from build123d import *

# Parameters (mm, degrees)
CUT_EXTRUDE_1_DEPTH      = 6
CUT_EXTRUDE_1_DEPTH_BACK = 6
SKETCH_2_W               = 26
SKETCH_2_H               = 10


with BuildPart() as part:
    # Sketch 1 → Revolve 1 (revolve)
    with BuildSketch(Plane.XY, mode=Mode.PRIVATE) as revolve_1_sk:
        Polygon((0, 0), (170, 0), (170, 10), (150, 10), (150, 15), (80, 15), (80, 20), (50, 20), (50, 12.5), (0, 12.5), align=None)
    revolve(revolve_1_sk.sketch.rotate(Axis((-10, 0, 0), (1, 0, 0)), 90), axis=Axis((-10, 0, 0), (1, 0, 0)))

    # Sketch 2 → Cut-Extrude 1 (cut, two sides: drawn at the far end of the back side and taken through both)
    with BuildSketch(Plane.XY.offset(-CUT_EXTRUDE_1_DEPTH_BACK)):
        with Locations((65, 20)):
            Rectangle(SKETCH_2_W, SKETCH_2_H)
    extrude(amount=CUT_EXTRUDE_1_DEPTH + CUT_EXTRUDE_1_DEPTH_BACK, mode=Mode.SUBTRACT)


solid = part.part
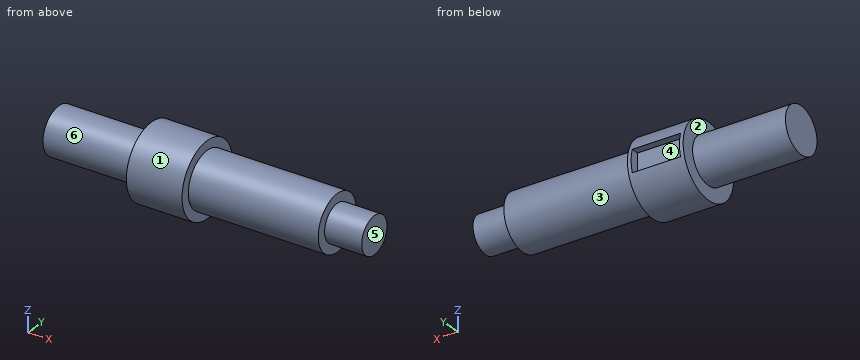
The listing builds one solid part. Answer for the finished solid, in the listing's coordinates (mm). Face numbers are marked on the shaded views. A direction names the side the tool comes from. Coordinates: 2 decimals unless noted, no trailing zeros. Write each loop counter-clockwise with the first axis right and the second up, starting at its lowest first coordinate (ties: lowest second). Pieces come first, ordered by that corner, then holes. Notation, with made-up numbers: (78.5, 86.5) - (86.5, 86.5) arc R23 cw to (86.5, 100.5) - close; hole circle Ø1 at (-14.75, 67). An arc over 180 degrees is marked (long way). Put each result on its own line as item: value.
1. Find the intervals of material crossed by line 1 along X through (y, z) = (-12, 3); line 2 along Z through (x, y) = (146.5, -0.5); line 3 along X through (y, z) = (18, -8), in increasing order. Write a range as from..to.
Answer sheet:
line 1: x = 0..150
line 2: z = -14.99..14.99
line 3: x = 50..80
2. The part is cut by section B-B on z = 0. Give the vertices of the cut face in (x, y), plus the area to 3 significant figures.
Answer sheet:
outline: (0, -12.5) - (50, -12.5) - (50, -20) - (80, -20) - (80, -15) - (150, -15) - (150, -10) - (170, -10) - (170, 10) - (150, 10) - (150, 15) - (80, 15) - (80, 20) - (78, 20) - (78, 15) - (52, 15) - (52, 20) - (50, 20) - (50, 12.5) - (0, 12.5) - close
area: 4,820 mm^2
3. Flat-ended cylindrical pins translate along their axes: pin 1 Ø1 at (x, y) = (147, 2.5) entering from +Z; pin 2 Ø1.5 at (y, z) = (-11.5, -13) entering from -X; pin 3 Ø6 at (x, z) = (67, 1) entering from +Y. Find the tip coordinate at first contact, or state that the pin passes through.
Answer sheet:
pin 1: stops at z = 14.87
pin 2: stops at x = 50
pin 3: stops at y = 15
4. The part is cut by section D-D on z = -8. Give the vertices of the cut face in (x, y).
Answer sheet:
outline: (0, -9.6) - (50, -9.6) - (50, -18.33) - (80, -18.33) - (80, -12.69) - (150, -12.69) - (150, -6) - (170, -6) - (170, 6) - (150, 6) - (150, 12.69) - (80, 12.69) - (80, 18.33) - (50, 18.33) - (50, 9.6) - (0, 9.6) - close
5. The part is cut by section C-C on x = 65. Give the vertices of the cut face in (y, z).
Answer sheet:
outline: (15, -6) - (15, 6) - (19.08, 6) arc R20 ccw (long way) to (19.08, -6) - close
6. The part is cut by section A-A on y = 0. Give the vertices of the cut face in (x, z), plus the area to 3 significant figures.
Answer sheet:
outline: (0, -12.5) - (50, -12.5) - (50, -20) - (80, -20) - (80, -15) - (150, -15) - (150, -10) - (170, -10) - (170, 10) - (150, 10) - (150, 15) - (80, 15) - (80, 20) - (50, 20) - (50, 12.5) - (0, 12.5) - close
area: 4,950 mm^2
7. Determine the mould class of the marked faces 4, 5 and 6 for opening direction Y: pulls with the +Y half, pulls with the -Y half, needs draft (parallel to the pull), parting line crosses it, or undercut.
Answer sheet:
face 4: pulls with the +Y half
face 5: needs draft
face 6: parting line crosses it
8. A tool of negligible diameter and unlimited length cuts with its end or side. For the marked faces 1, 2 and 3, from which of +Z, -Z, +X, -X, +Y, -Y can it reach the whole face along a straight path? Write none if from no direction.
Answer sheet:
face 1: +X, -X
face 2: -X
face 3: +X
